Geometry check sheet. Reference: the model listing, model coordinates, mm. Round coordinates to 2 decimals unless told otherwise and drop trailing zeros. Order: outer loops, then holes, each group sorted by start corner. A loop starts at its lowest first (then second) coordinate and runs counter-clockwise, first axis right, second up. Notation, with made-up numbers: (75.25, -5) -> (125.25, -5) arc R16 cw to (125.25, 14) -> close; hole circle Ø3 at (62.25, -8.5). An arc over 180 degrees is marked (long way). Use a Markdown table: item, result. Add a question column.
Item 1: Sectioned sample at D-D, the plane y = -89. Record the cut outline in (x, z) (3 decimals), and give its area (3 significant figures).
Item 2: Gauge pin test, flat ends, axial feed: pin 1 Ø1 at (x, z) = (-178, -1) entering from +Y; pin 2 Ø1.6 at (x, z) = (-191, -2.5) entering from -Y. Record the tip position at first contact, or that the pin passes through.
Item 3: Sectioned sample at A-A, the plane x = 173. Record the cut outline in (y, z) (1 decimal), and give its area (3 significant figures).
Item 4: Sectioned sample at C-C, the plane x = -192.5. Record the cut outline in (y, z) (1 decimal).
Item 5: Sectioned sample at B-B, the plane z = -2. State how many separate pieces and enclosed holes the cut face has, and give its area (3 significant figures).
Item 6: Material ranges on probe 1 along Y at (x, z) = (166, -2.45); probe 2 along Y at (x, z) = (-188.5, -2.05); probe 3 along Y at (x, z) = (8, -0.55), recorded low to high. Write a range as [from, to].
from build123d import *

# Parameters (mm, degrees)
SKETCH1_W               = 475.54896
SKETCH1_H               = 657.23516
BASE_FLANGE1_DEPTH      = 3.175
CUT_EXTRUDE1_DEPTH      = 406.63074076
CUT_EXTRUDE1_DEPTH_BACK = 406.63074076
SKETCH2_W               = 60.325
SKETCH2_H               = 3.175
SKETCH3_W               = 107.287119944
SKETCH3_H               = 35.306
SKETCH3_W_2             = 35.306
SKETCH3_H_2             = 127.472499944
BOSS_EXTRUDE1_DEPTH     = 3.175


# Sheet-metal steps are written as plain solids
with BuildPart() as part:
    # Sketch1 → Base-Flange1 (new body)
    with BuildSketch(Plane.XY):
        Rectangle(SKETCH1_W, SKETCH1_H)
    extrude(amount=-BASE_FLANGE1_DEPTH)

    # Sketch2 → Cut-Extrude1 (cut, two sides: drawn at the far end of the back side and taken through both)
    with BuildSketch(Plane.XY.offset(-CUT_EXTRUDE1_DEPTH_BACK)):
        with Locations((-186.97448, 220.13672)):
            Rectangle(SKETCH2_W, SKETCH2_H)
        with Locations((186.97448, -220.13672)):
            Rectangle(SKETCH2_W, SKETCH2_H)
        with Locations((186.97448, 220.13672)):
            Rectangle(SKETCH2_W, SKETCH2_H)
        with Locations((-186.97448, -220.13672)):
            Rectangle(SKETCH2_W, SKETCH2_H)
        with Locations((-186.97448, 0)):
            Rectangle(SKETCH2_W, SKETCH2_H)
        with Locations((186.97448, -110.06836)):
            Rectangle(SKETCH2_W, SKETCH2_H)
        with Locations((-186.97448, -110.06836)):
            Rectangle(SKETCH2_W, SKETCH2_H)
        with Locations((-186.97448, 110.06836)):
            Rectangle(SKETCH2_W, SKETCH2_H)
        with Locations((186.97448, 0)):
            Rectangle(SKETCH2_W, SKETCH2_H)
        with Locations((186.97448, 110.06836)):
            Rectangle(SKETCH2_W, SKETCH2_H)
    extrude(amount=CUT_EXTRUDE1_DEPTH + CUT_EXTRUDE1_DEPTH_BACK, mode=Mode.SUBTRACT)

    # Sketch3 → Boss-Extrude1 (add)
    with BuildSketch(Plane.XY):
        with Locations((184.130920028, 346.27058)):
            Rectangle(SKETCH3_W, SKETCH3_H)
        with Locations((-255.42748, 264.881330028)):
            Rectangle(SKETCH3_W_2, SKETCH3_H_2)
        with Locations((-255.42748, -264.881330028)):
            Rectangle(SKETCH3_W_2, SKETCH3_H_2)
        with Locations((184.130920028, -346.27058)):
            Rectangle(SKETCH3_W, SKETCH3_H)
    extrude(amount=-BOSS_EXTRUDE1_DEPTH)


solid = part.part
Found:
| question | item | result |
|---|---|---|
| 1 | outline | (-237.774, -3.175) -> (237.774, -3.175) -> (237.774, 0) -> (-237.774, 0) -> close |
| 1 | area | 1,510 mm2 |
| 2 | pin 1 | stops at y = 328.62 |
| 2 | pin 2 | stops at y = -328.62 |
| 3 | outline | (-363.9, -3.2) -> (-221.7, -3.2) -> (-221.7, 0) -> (-363.9, 0) -> close; (-218.5, -3.2) -> (-111.7, -3.2) -> (-111.7, 0) -> (-218.5, 0) -> close; (-108.5, -3.2) -> (-1.6, -3.2) -> (-1.6, 0) -> (-108.5, 0) -> close; (1.6, -3.2) -> (108.5, -3.2) -> (108.5, 0) -> (1.6, 0) -> close; (111.7, -3.2) -> (218.5, -3.2) -> (218.5, 0) -> (111.7, 0) -> close; (221.7, -3.2) -> (363.9, -3.2) -> (363.9, 0) -> (221.7, 0) -> close |
| 3 | area | 2,260 mm2 |
| 4 | outline | (-328.6, -3.2) -> (-221.7, -3.2) -> (-221.7, 0) -> (-328.6, 0) -> close; (-218.5, -3.2) -> (-111.7, -3.2) -> (-111.7, 0) -> (-218.5, 0) -> close; (-108.5, -3.2) -> (-1.6, -3.2) -> (-1.6, 0) -> (-108.5, 0) -> close; (1.6, -3.2) -> (108.5, -3.2) -> (108.5, 0) -> (1.6, 0) -> close; (111.7, -3.2) -> (218.5, -3.2) -> (218.5, 0) -> (111.7, 0) -> close; (221.7, -3.2) -> (328.6, -3.2) -> (328.6, 0) -> (221.7, 0) -> close |
| 5 | separate pieces | 1 |
| 5 | enclosed holes | 10 |
| 5 | area | 327,000 mm2 |
| 6 | probe 1 | y = [-363.92, -221.72], [-218.55, -111.66], [-108.48, -1.59], [1.59, 108.48], [111.66, 218.55], [221.72, 363.92] |
| 6 | probe 2 | y = [-328.62, -221.72], [-218.55, -111.66], [-108.48, -1.59], [1.59, 108.48], [111.66, 218.55], [221.72, 328.62] |
| 6 | probe 3 | y = [-328.62, 328.62] |
